The listing builds one solid part. Answer for the finished solid, in the listing's coordinates (mm). A direction names the side the tool comes from. Round coordinates to 2 decimals unless told otherwise and drop trailing zeros. Write each loop counter-clockwise with the first axis right and the second up, starting at its lowest first coordinate (ties: lowest second). Pieces come first, ordered by that corner, then holes. Notation, with made-up numbers: (-36, 16) - (-31, 16) arc R17 ccw to (-31, 35) - close; hole circle Ø7 at (-17.75, -37.75). An arc over 180 degrees is marked (long way). Return JSON: item names as keys, results as strings. Group by question number.
(1) Section C-C, the plane x = 16 is taken. Write down the section's boundary in (y, z).
(2) Section D-D, the plane z = 35 is taken. Write down the section's boundary in (x, y).
(3) Find the intervals of material crossed by line 1 along Z through (x, y) = (-37, -24); line 2 along Y through (x, z) = (-38.5, 7.5); line 3 along Z through (x, y) = (26.5, -33), in increasing order. Write a range as [from, to].
(4) Which of the six approach directions +Z, -Z, +X, -X, +Y, -Y give full straight-line access (tool end or side, diameter ignored) to faces 1 (the flat face through (4, -12, 40.545)), 2 (the flat face through (26, -15, 28)), 3 (the flat face through (-17.69, -30, 18))?
(5) Section B-B, the plane z = 27.5 is taken. Write down the section's boundary in (x, y), then the cut area to 3 significant figures.
(6) Each of these flat-tipped pins is pushed along its axis until it touches: pin 1 (15 mm diameter, centred on x = -38, y = -24.5, fed in from +Z); pin 2 (4 mm diameter, centred on x = -40.5, z = -11, fed in from +Y); pin 3 (5 mm diameter, centred on y = -12, z = 11, fed in from -X); pin 4 (10 mm diameter, centred on y = -17, z = 14.5, fed in from -X). Where does it stop, or does it pass through?
(7) Section A-A, the plane y = -25 is taken. Write down the section's boundary in (x, z), then the cut area to 4 significant figures.
```python
from build123d import *

# Parameters (mm, degrees)
F1_DEPTH = 45
F3_DEPTH = 30
F5_DEPTH = 30


with BuildPart() as f1:
    # F0 (on Front) → F1 (new body)
    with BuildSketch(Plane.XZ):
        Polygon((-17.689841, 40.544534), (-62.689841, -4.455466), (-62.689841, -19.455466), (37.310159, -19.455466), (37.310159, -4.455466), (37.310159, 40.544534), (-2.689841, 40.544534), align=None)
    extrude(amount=F1_DEPTH)

    # F2 (on face) → F3 (cut)
    with BuildSketch(Plane.XZ.offset(45)):
        Polygon((-17.689841, -4.455466), (-17.689841, 40.544534), (-62.689841, -4.455466), align=None)
    extrude(amount=-F3_DEPTH, mode=Mode.SUBTRACT)

    # F4 (on face) → F5 (cut)
    with BuildSketch(Plane.XZ.offset(45)):
        Polygon((37.310159, 40.544534), (-2.689841, 40.544534), (37.310159, -4.455466), align=None)
    extrude(amount=-F5_DEPTH, mode=Mode.SUBTRACT)


solid = f1.part
```
Working result:
{
 "1": {"outline": "(-45, -19.46) - (0, -19.46) - (0, 40.54) - (-15, 40.54) - (-15, 19.52) - (-45, 19.52) - close"},
 "2": {"outline": "(-23.23, -15) - (-17.69, -15) - (-17.69, -45) - (2.24, -45) - (2.24, -15) - (37.31, -15) - (37.31, 0) - (-23.23, 0) - close"},
 "3": {"line 1": "z = [-19.46, -4.46]", "line 2": "y = [-15, 0]", "line 3": "z = [-19.46, 7.71]"},
 "4": {"face 1": "+Z, +X, -X, +Y, -Y", "face 2": "+Z, +X, -Y", "face 3": "+Z, -X, -Y"},
 "5": {"outline": "(-30.73, -15) - (-17.69, -15) - (-17.69, -45) - (8.91, -45) - (8.91, -15) - (37.31, -15) - (37.31, 0) - (-30.73, 0) - close", "area": "1,820 mm^2"},
 "6": {"pin 1": "stops at z = -4.46", "pin 2": "stops at y = 0", "pin 3": "stops at x = -49.73", "pin 4": "stops at x = -48.32"},
 "7": {"outline": "(-62.69, -19.46) - (37.31, -19.46) - (37.31, -4.46) - (-2.69, 40.54) - (-17.69, 40.54) - (-17.69, -4.46) - (-62.69, -4.46) - close", "area": "3,075 mm^2"}
}
